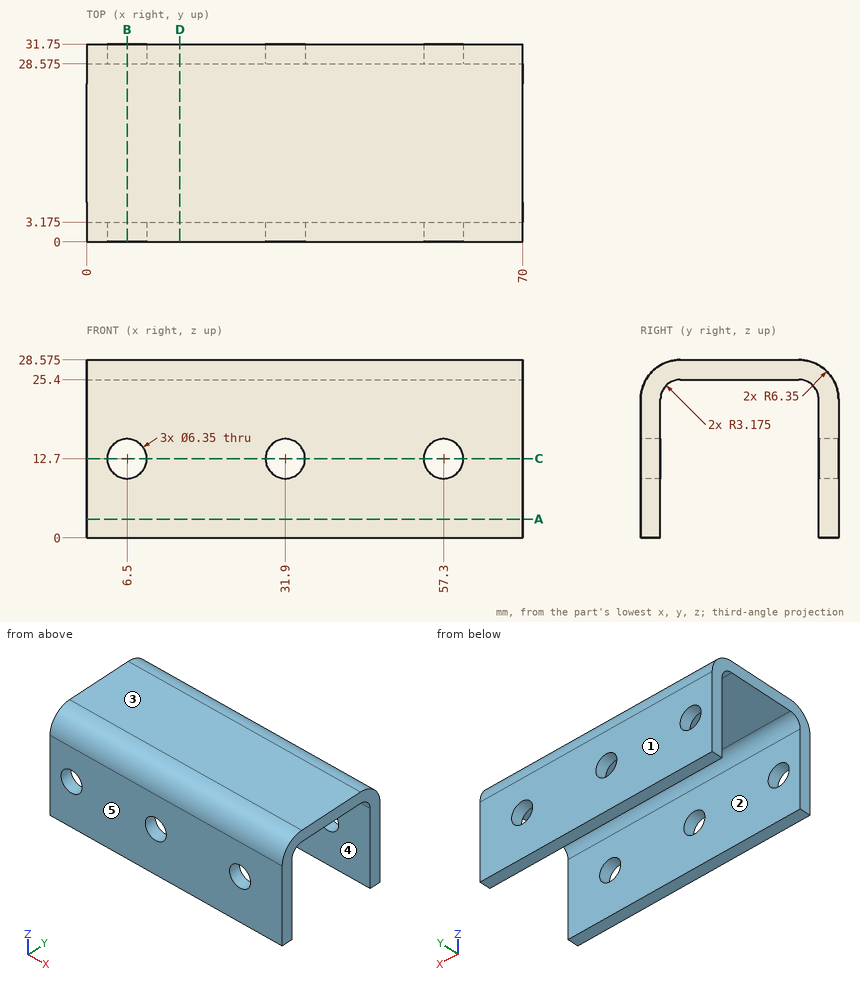
Check sheet for the drawn part. Datum: minimum x, y, z corner. Units: mm. A direction names the side the tool comes from. Give positions to 0.01 mm unless a question says otherwise; leave off trailing zeros. Order: outer loops, then holes, each group sorted by start corner. A loop starts at its lowest first (then second) coordinate and runs counter-clockwise, first axis right, second up.
1. Depth check by flat-ended pin: pin 1 (10 mm diameter, centred on y = 21, z = 4, fed in from +X); pin 2 (2 mm diameter, centred on x = 35, z = 25, fed in from -Y); pin 3 (5.5 mm diameter, centred on x = 30.5, y = 18, fed in from -Z). Enter the tip coordinate at first touch or a pass-through.
Completed:
pin 1: passes through
pin 2: stops at y = 0.25
pin 3: stops at z = 25.4
2. Scan lines: line 1 (Y direction, x = 39.5, z = 17.75) (3 decimals); line 2 (Z direction, x = 30, y = 21.5) (3 decimals); line 3 (Z direction, x = 57, y = 2). Record each from-to range of solid material in increasing order.
Completed:
line 1: y = 0 to 3.175, 28.575 to 31.75
line 2: z = 25.4 to 28.575
line 3: z = 0 to 9.54, 15.86 to 26.85
3. Sectioned sample at A-A (z = 3). Record the boundary of the cut face in (x, y) (3 decimals).
Completed:
outline: (0, 0) - (70, 0) - (70, 3.175) - (0, 3.175) - close; (0, 28.575) - (70, 28.575) - (70, 31.75) - (0, 31.75) - close
4. Access from +Z, -Z, +X, -X, +Y, -Y to the whole of each face (thin tool, end or side, straight path). Record for the marked faces 1 and 2.
Completed:
face 1: +Z, -Z, +X, -X, +Y
face 2: -Z, +X, -X
5. Sectioned sample at D-D (x = 15). Record the boundary of the cut face in (y, z) (3 decimals), then the cut area to 3 significant figures.
Completed:
outline: (0, 0) - (3.175, 0) - (3.175, 22.225) arc R3.175 cw to (6.35, 25.4) - (25.4, 25.4) arc R3.175 cw to (28.575, 22.225) - (28.575, 0) - (31.75, 0) - (31.75, 22.225) arc R6.35 ccw to (25.4, 28.575) - (6.35, 28.575) arc R6.35 ccw to (0, 22.225) - close
area: 249 mm2
6. Sectioned sample at B-B (x = 6.5). Record the boundary of the cut face in (y, z) (3 decimals).
Completed:
outline: (0, 0) - (3.175, 0) - (3.175, 9.525) - (0, 9.525) - close; (0, 15.875) - (3.175, 15.875) - (3.175, 22.225) arc R3.175 cw to (6.35, 25.4) - (25.4, 25.4) arc R3.175 cw to (28.575, 22.225) - (28.575, 15.875) - (31.75, 15.875) - (31.75, 22.225) arc R6.35 ccw to (25.4, 28.575) - (6.35, 28.575) arc R6.35 ccw to (0, 22.225) - close; (28.575, 0) - (31.75, 0) - (31.75, 9.525) - (28.575, 9.525) - close
7. Draft check along Y on the marked faces 3, 4 and 5. Enter one of: pulls with the +Y half, pulls with the -Y half, needs draft (parallel to the pull), parting line crosses it, or undercut.
Completed:
face 3: needs draft
face 4: undercut
face 5: pulls with the -Y half
8. Sectioned sample at C-C (z = 12.7). State how many separate pieces and enclosed holes the cut face has, then the cut area to 3 significant figures.
Completed:
separate pieces: 8
enclosed holes: 0
area: 324 mm2
